Design review of the part built by this model. Coordinates are the model's own, in mm. A direction names the side the tool comes from. Round coordinates to 2 decimals unless told otherwise and drop trailing zeros. Loops run counter-clockwise (first coordinate to the right, second up) from the corner with the lowest first, then second, coordinate; pieces in that order, holes last. Notation, with made-up numbers: M 39.25,20 L 89.25,20 A13 cw 89.25,29 Z; hole C -22.5,78.5 d5. An arc over 180 degrees is marked long. Use a Markdown table: item, result.
from build123d import *

# Parameters (mm, degrees)
ESBO_O2_R                = 1.6
RESSALTO_EXTRUS_O1_DEPTH = 1.52
ESBO_O3_W                = 9.096465254
ESBO_O3_H                = 14.507430643
RESSALTO_EXTRUS_O2_DEPTH = 11
ESBO_O4_W                = 2.45
ESBO_O4_H                = 38.5
ESBO_O4_H_2              = 46
RESSALTO_EXTRUS_O3_DEPTH = 8.4
CORTE_EXTRUS_O1_DEPTH    = 12
ESBO_O6_R                = 3.548232627
ESBO_O6_R_2              = 1
CORTE_EXTRUS_O2_DEPTH    = 12
FILETE1_R                = 1
FILETE2_R                = 0.5
ESBO_O7_W                = 12.140382315
ESBO_O7_H                = 16.18717642
RESSALTO_EXTRUS_O4_DEPTH = 10.8
CORTE_EXTRUS_O3_DEPTH    = 10
ESBO_O10_W               = 10.15094297
ESBO_O10_H               = 41.419472655
RESSALTO_EXTRUS_O5_DEPTH = 7
FILETE3_R                = 1
ESBO_O11_W               = 11.15094297
ESBO_O11_H               = 42.419472655
RESSALTO_EXTRUS_O6_DEPTH = 3


with BuildPart() as part:
    # Esboço2 → Ressalto-extrusão1 (new body)
    with BuildSketch(Plane.XY):
        with BuildLine():
            Line((26.8, -30.283131706), (25.193131706, -31.89))
            Line((25.193131706, -31.89), (13.76, -31.89))
            Line((13.76, -31.89), (11.5, -34.15))
            Line((11.5, -34.15), (-21.7, -34.15))
            Line((-21.7, -34.15), (-23.96, -31.89))
            Line((-23.96, -31.89), (-25.8, -31.89))
            ThreePointArc((-25.8, -31.89), (-26.507106781, -31.597106781), (-26.8, -30.89))
            Line((-26.8, -30.89), (-26.8, 33.15))
            ThreePointArc((-26.8, 33.15), (-26.507106781, 33.857106781), (-25.8, 34.15))
            Line((-25.8, 34.15), (25.8, 34.15))
            ThreePointArc((25.8, 34.15), (26.507106781, 33.857106781), (26.8, 33.15))
            Line((26.8, 33.15), (26.8, -30.283131706))
        make_face()
        with Locations((-24, 18.91)):
            Circle(ESBO_O2_R, mode=Mode.SUBTRACT)
        with Locations((24.26, 18.91)):
            Circle(ESBO_O2_R, mode=Mode.SUBTRACT)
        with Locations((-18.92, -31.89)):
            Circle(ESBO_O2_R, mode=Mode.SUBTRACT)
        with Locations((9.02, -31.89)):
            Circle(ESBO_O2_R, mode=Mode.SUBTRACT)
    extrude(amount=RESSALTO_EXTRUS_O1_DEPTH)

    # Esboço3 → Ressalto-extrusão2 (add)
    with BuildSketch(Plane.XY.offset(1.52)):
        with Locations((-19.138446447, 28.272429058)):
            Rectangle(ESBO_O3_W, ESBO_O3_H)
    extrude(amount=RESSALTO_EXTRUS_O2_DEPTH)

    # Esboço4 → Ressalto-extrusão3 (add)
    with BuildSketch(Plane.XY.offset(1.52)):
        with Locations((-23.575, -10.64)):
            Rectangle(ESBO_O4_W, ESBO_O4_H)
        with Locations((23.575, -6.89)):
            Rectangle(ESBO_O4_W, ESBO_O4_H_2)
    extrude(amount=RESSALTO_EXTRUS_O3_DEPTH)

    # Esboço5 → Corte-extrusão1 (cut)
    with BuildSketch(Plane.XZ.offset(-21.018713736)):
        with BuildLine():
            Line((-14.59021382, 7.52), (-14.59021382, 12.52))
            Line((-14.59021382, 12.52), (-23.686679074, 12.52))
            Line((-23.686679074, 12.52), (-23.686679074, 7.52))
            ThreePointArc((-23.686679074, 7.52), (-19.138446447, 12.068232627), (-14.59021382, 7.52))
        make_face()
    extrude(amount=-CORTE_EXTRUS_O1_DEPTH, mode=Mode.SUBTRACT)

    # Esboço6 → Corte-extrusão2 (cut)
    with BuildSketch(Plane.XZ.offset(-35.526144379)):
        with Locations(Location((-19.138446447, 7.52, 0), (0, 0, 270))):
            Circle(ESBO_O6_R)
        with Locations(Location((-19.138446447, 7.52, 0), (0, 0, 270))):
            Circle(ESBO_O6_R_2, mode=Mode.SUBTRACT)
    extrude(amount=CORTE_EXTRUS_O2_DEPTH, mode=Mode.SUBTRACT)

    # Filete1
    filete1_edges = [part.edges().sort_by_distance(p)[0] for p in [
        (-19.138446447, 35.526144379, 8.52),
    ]]
    fillet(filete1_edges, radius=FILETE1_R)

    # Filete2
    filete2_edges = [part.edges().sort_by_distance(p)[0] for p in [
        (-23.686679074, 34.272429057, 12.52),
        (-14.59021382, 34.272429057, 12.52),
    ]]
    fillet(filete2_edges, radius=FILETE2_R)

    # Esboço7 → Ressalto-extrusão4 (add)
    with BuildSketch(Plane.XY.offset(1.52)):
        with Locations((11.10014829, 32.59935696)):
            Rectangle(ESBO_O7_W, ESBO_O7_H)
    extrude(amount=RESSALTO_EXTRUS_O4_DEPTH)

    # Esboço9 → Corte-extrusão3 (cut)
    with BuildSketch(Plane(origin=(0, 40.69294517, 0), x_dir=(1, 0, 0), z_dir=(0, 1, 0))):
        with BuildLine():
            Line((6.729957133, -2.72), (15.470339448, -2.72))
            ThreePointArc((15.470339448, -2.72), (15.823892839, -2.866446609), (15.970339448, -3.22))
            Line((15.970339448, -3.22), (15.970339448, -8.912893219))
            ThreePointArc((15.970339448, -8.912893219), (15.932279214, -9.104234935), (15.823892839, -9.266446609))
            Line((15.823892839, -9.266446609), (14.116786058, -10.973553391))
            ThreePointArc((14.116786058, -10.973553391), (13.954574383, -11.081939766), (13.763232667, -11.12))
            Line((13.763232667, -11.12), (8.437063914, -11.12))
            ThreePointArc((8.437063914, -11.12), (8.245722198, -11.081939766), (8.083510523, -10.973553391))
            Line((8.083510523, -10.973553391), (6.376403742, -9.266446609))
            ThreePointArc((6.376403742, -9.266446609), (6.268017366, -9.104234935), (6.229957133, -8.912893219))
            Line((6.229957133, -8.912893219), (6.229957133, -3.22))
            ThreePointArc((6.229957133, -3.22), (6.376403742, -2.866446609), (6.729957133, -2.72))
        make_face()
        with BuildLine():
            Line((13.80014829, -8.17), (8.40014829, -8.17))
            ThreePointArc((8.40014829, -8.17), (8.188016256, -8.082132034), (8.10014829, -7.87))
            Line((8.10014829, -7.87), (8.10014829, -5.97))
            ThreePointArc((8.10014829, -5.97), (8.188016256, -5.757867966), (8.40014829, -5.67))
            Line((8.40014829, -5.67), (13.80014829, -5.67))
            ThreePointArc((13.80014829, -5.67), (14.012280325, -5.757867966), (14.10014829, -5.97))
            Line((14.10014829, -5.97), (14.10014829, -7.87))
            ThreePointArc((14.10014829, -7.87), (14.012280325, -8.082132034), (13.80014829, -8.17))
        make_face(mode=Mode.SUBTRACT)
    extrude(amount=-CORTE_EXTRUS_O3_DEPTH, mode=Mode.SUBTRACT)

    # Esboço10 → Ressalto-extrusão5 (add)
    with BuildSketch(Plane.XY.offset(1.52)):
        with Locations((-9.018025228, -5.927819482)):
            Rectangle(ESBO_O10_W, ESBO_O10_H)
    extrude(amount=RESSALTO_EXTRUS_O5_DEPTH)

    # Filete3
    filete3_edges = [part.edges().sort_by_distance(p)[0] for p in [
        (-3.942553743, -5.927819482, 8.52),
        (-9.018025228, 14.781916846, 8.52),
        (-14.093496713, -5.927819482, 8.52),
        (-9.018025228, -26.637555809, 8.52),
    ]]
    fillet(filete3_edges, radius=FILETE3_R)

    # Esboço11 → Ressalto-extrusão6 (add)
    with BuildSketch(Plane.XY.offset(1.52)):
        with Locations((-9.018025228, -5.927819482)):
            Rectangle(ESBO_O11_W, ESBO_O11_H)
    extrude(amount=RESSALTO_EXTRUS_O6_DEPTH)


solid = part.part
1. Insertion check: pin 1 (4 mm diameter, centred on x = 20.5, z = 4, fed in from +Y); pin 2 (1.5 mm diameter, centred on x = -6.5, z = 6.5, fed in from -Y); pin 3 (5 mm diameter, centred on x = 4.5, y = 26.5, fed in from -Z); pin 4 (3.5 mm diameter, centred on x = 9, y = 36, fed in from -Z). Each pin has a flat end and moves straight along its axis. Give the tip position at first contact, or say it passes through.
Check values:
| item | result |
|---|---|
| pin 1 | stops at y = 16.11 |
| pin 2 | stops at y = -26.64 |
| pin 3 | stops at z = 0 |
| pin 4 | stops at z = 1.52 |
2. Take a section at C-C on x = 0.5. Give the boundary of the cut face in (y, z).
Check values:
| item | result |
|---|---|
| outline | M -34.15,0 L 34.15,0 L 34.15,1.52 L -34.15,1.52 Z |
3. Wall thickness on line 1 along Z through (x, y) = (13.5, 33.5); line 2 along X through (y, z) = (-1.5, 7.5); line 3 along X through (y, z) = (10, 7.5): over which ranges is each line inside the solid? List them lowest first. Write a range as from..to.
Check values:
| item | result |
|---|---|
| line 1 | z = 0..2.72, 5.67..8.17, 11.12..12.32 |
| line 2 | x = -24.8..-22.35, -14.09..-3.94, 22.35..24.8 |
| line 3 | x = -14.09..-3.94, 22.35..24.8 |
4. The part is to be moulded in two halves that separate along X. For faces 1 (the face through (-24.208, 20.496, 0.749)), 2 (the face through (-22.81, -33.04, 0.75)), 3 (the face through (-9, -27.138, 3)), 4 (the face through (24, -7, 9.92)), say which applies: pulls with the +X half, pulls with the -X half, needs draft (parallel to the pull), parting line crosses it, or undercut.
Check values:
| item | result |
|---|---|
| face 1 | undercut |
| face 2 | pulls with the -X half |
| face 3 | undercut |
| face 4 | needs draft |
5. Machinability: for faces 5 (the face through (-3.943, -6, 6)), 6 (the face through (-22.35, -11, 6)), 7 (the face through (-25, -31.89, 1)), which of the approach directions +Z, -Z, +X, -X, +Y, -Y give a long, thin tool a straight path to every point of the face, cutting with its end or side? Answer none if there is none.
Check values:
| item | result |
|---|---|
| face 5 | +Z, +Y, -Y |
| face 6 | +Z, -Y |
| face 7 | +Z, -Z, -X, -Y |
6. Take a section at B-B on y = -13. Give the boundary of the cut face in (x, z).
Check values:
| item | result |
|---|---|
| outline | M -26.8,0 L 26.8,0 L 26.8,1.52 L 24.8,1.52 L 24.8,9.92 L 22.35,9.92 L 22.35,1.52 L -3.44,1.52 L -3.44,4.52 L -3.94,4.52 L -3.94,7.52 A1 ccw -4.94,8.52 L -13.09,8.52 A1 ccw -14.09,7.52 L -14.09,4.52 L -14.59,4.52 L -14.59,1.52 L -22.35,1.52 L -22.35,9.92 L -24.8,9.92 L -24.8,1.52 L -26.8,1.52 Z |
7. Take a section at A-A on y = 13. Give the boundary of the cut face in (x, z), and give its area (3 significant figures).
Check values:
| item | result |
|---|---|
| outline | M -26.8,0 L 26.8,0 L 26.8,1.52 L 24.8,1.52 L 24.8,9.92 L 22.35,9.92 L 22.35,1.52 L -3.44,1.52 L -3.44,4.52 L -3.94,4.52 L -3.94,7.52 A1 ccw -4.94,8.52 L -13.09,8.52 A1 ccw -14.09,7.52 L -14.09,4.52 L -14.59,4.52 L -14.59,1.52 L -26.8,1.52 Z |
| area | 176 mm² |
8. Take a section at D-D on y = -28.5. Give the boundary of the cut face in (x, z), and give its area (3 significant figures).
Check values:
| item | result |
|---|---|
| outline | M -26.8,0 L 26.8,0 L 26.8,1.52 L 24.8,1.52 L 24.8,9.92 L 22.35,9.92 L 22.35,1.52 L -22.35,1.52 L -22.35,9.92 L -24.8,9.92 L -24.8,1.52 L -26.8,1.52 Z |
| area | 123 mm² |
